The listing builds one solid part. Answer for the finished solid, in the listing's coordinates (mm). Give positions to 0.01 mm unless a question says otherwise; leave off trailing zeros. Order: outer loops, then holes, each group sorted by start corner. A loop starts at its lowest first (then second) coordinate and runs counter-clockwise, first axis right, second up. Notation, with made-up numbers: M 56,-1.5 L 88,-1.5 A7 cw 88,2.5 Z; hole C -37,64.25 d10. An arc over 180 degrees is marked long. Answer as a JSON object with one key per item and string values. Group by question number.
```python
from build123d import *

# Parameters (mm, degrees)
SKETCH1_R           = 45
SKETCH1_R_2         = 40
BOSS_EXTRUDE1_DEPTH = 22
CHAMFER1_SIZE       = 2
FILLET1_R           = 1


with BuildPart() as part:
    # Sketch1 → Boss-Extrude1 (new body)
    with BuildSketch(Plane.XY):
        Circle(SKETCH1_R)
        Circle(SKETCH1_R_2, mode=Mode.SUBTRACT)
    extrude(amount=BOSS_EXTRUDE1_DEPTH)

    # Chamfer1
    chamfer1_edges = [part.edges().sort_by_distance(p)[0] for p in [
        (-45, 0, 0),
    ]]
    chamfer(chamfer1_edges, length=CHAMFER1_SIZE)

    # Fillet1
    fillet1_edges = [part.edges().sort_by_distance(p)[0] for p in [
        (-45, 0, 2),
        (-43, 0, 0),
        (-40, 0, 0),
    ]]
    fillet(fillet1_edges, radius=FILLET1_R)


solid = part.part
```
Item 1: Determine the mould class of faces 1 (the cylindrical face through (-8.67, -39.05, 11.35)), 2 (the conical face through (40.1, -16.6, 0.4)), 3 (the flat face through (-30.2, -26.5, 22)) for opening direction X: released by +X, released by -X, zero draft, split by the parting line, or undercut.
Item 2: Flat-ended cylindrical pins translate along their axes: P1, Ø2, axis at x = 9.5, z = 17.5, coming from the -Y side; P2, Ø3, axis at x = -17.5, z = 9, coming from the +Y side; P3, Ø10, axis at x = 18.5, z = 8.5, coming from the +Y side. Find the tip coordinate at first contact, or state that the pin passes through.
Item 3: Consider probe 1 along Y at (x, z) = (0, 17.75); probe 2 along X at (y, z) = (-1, 12); probe 3 along Y at (x, z) = (6.5, 14.75). Determine where each line is inside the solid, lowest interval first. Write a range as from..to.
Item 4: Section A-A (z = 19.25) is taken. Determine the outline of the cut face in (x, y).
Values found:
{
 "1": {"face 1": "undercut", "face 2": "split by the parting line", "face 3": "zero draft"},
 "2": {"P1": "stops at y = -44.19", "P2": "stops at y = 42.06", "P3": "stops at y = 42.93"},
 "3": {"probe 1": "y = -45..-40, 40..45", "probe 2": "x = -44.99..-39.99, 39.99..44.99", "probe 3": "y = -44.53..-39.47, 39.47..44.53"},
 "4": {"outline": "C 0,0 d90; hole C 0,0 d80"}
}
